from build123d import *

# Parameters (mm, degrees)
F0_R     = 50.8
F1_DEPTH = 7.62
F2_R     = 38.1
F3_DEPTH = 124.206
F3_TAPER = 20
F4_R     = 2.3749
F4_R_2   = 2.38125
F5_DEPTH = 25.4


with BuildPart() as f1:
    # F0 (on Top) → F1 (new body)
    with BuildSketch(Plane.XY):
        Circle(F0_R)
    extrude(amount=F1_DEPTH)

    # F2 (on face) → F3 (join)
    with BuildSketch(Plane.XY.offset(7.62)):
        Circle(F2_R)
    extrude(amount=F3_DEPTH, taper=F3_TAPER)

    # F4 (on Top) → F5 (cut)
    with BuildSketch(Plane.XY):
        with Locations((-25.4, -38.1)):
            Circle(F4_R)
        with Locations((25.4, -38.1)):
            Circle(F4_R_2)
        with Locations((-25.4, 38.1)):
            Circle(F4_R)
        with Locations((25.4, 38.1)):
            Circle(F4_R_2)
    extrude(amount=F5_DEPTH, mode=Mode.SUBTRACT)


solid = f1.part
Could you check a few things on this model? Use its own coordinates, in mm. A direction names the side the tool comes from. Give positions to 0.01 mm unless a question says otherwise; leave off trailing zeros. Order: outer loops, then holes, each group sorted by start corner. A loop starts at its lowest first (then second) coordinate and runs counter-clockwise, first axis right, second up.
Item 1: For faces 1 (the face through (-11.012, -49.592, 3.757)), 2 (the face through (7, 38, 7.62)), which set-ups out of +Z, -Z, +X, -X, +Y, -Y let a thin tool reach every point of the face, with its end or its side?
Item 2: If we mould it in two halves opening along X, with no side actions, what happens to faces 3 (the face through (-11.55, -8.85, 72.32)), 4 (the face through (-24.304, 35.993, 3.757)), 5 (the face through (-1, 1, 0))? For each: pulls with the +X half, pulls with the -X half, needs draft (parallel to the pull), parting line crosses it, or undercut.
Item 3: If we section it at B-B, the plane x = -41: Write out the boundary of the cut face in (y, z).
Item 4: I'm going to push flat-ended pins straight in: pin 1 (12 mm diameter, centred on y = -10, z = 56, fed in from -X); pin 2 (6 mm diameter, centred on x = 25.4, y = -38.1, fed in from +Z); pin 3 (10 mm diameter, centred on y = 4.5, z = 43, fed in from -X). Where does each tip first touch, or does it pass through?
Item 5: I need wall thicknesses on line 1 (Y direction, x = -25, z = 2); line 2 (X direction, y = -38.1, z = 2.5); line 3 (X direction, y = 38, z = 5). Which ranges of each line are inside material? Lowest first, please.
Item 6: If we section it at C-C, the plane z = 30: Write out the boundary of the cut face in (x, y).
Item 7: If we section it at A-A, the plane z = 56: Write out the boundary of the cut face in (x, y), plus the area to 3 significant figures.
Values:
1. face 1: +Z, -Z
1. face 2: +Z
2. face 3: parting line crosses it
2. face 4: undercut
2. face 5: needs draft
3. outline: (-29.99, 0) - (29.99, 0) - (29.99, 7.62) - (-29.99, 7.62) - close
4. pin 1: stops at x = -21.3
4. pin 2: stops at z = 7.62
4. pin 3: stops at x = -26.79
5. line 1: y = -44.22 to -40.44, -35.76 to 35.76, 40.44 to 44.22
5. line 2: x = -33.6 to -27.77, -23.03 to 23.02, 27.78 to 33.6
5. line 3: x = -33.71 to -27.77, -23.03 to 23.02, 27.78 to 33.71
6. outline: circle Ø59.91 at (0, 0)
7. outline: circle Ø40.98 at (0, 0)
7. area: 1,320 mm2
